from build123d import *

# Parameters (mm, degrees)
EXTRUDE_1_DEPTH     = 30
CUT_EXTRUDE_2_DEPTH = 60.044241887
EXTRUDE_2_DEPTH     = 30
FILLET_2_R          = 10
FILLET_3_R          = 10
SKETCH_6_R          = 1.65
CUT_EXTRUDE_3_DEPTH = 60.044242053
FILLET_4_R          = 2
FILLET_6_R          = 5


with BuildPart() as part:
    # 草图2 → 凸台-拉伸1 (new body)
    with BuildSketch(Plane.XY):
        with BuildLine():
            Line((-22, 40.85), (-22, -8.75))
            ThreePointArc((-22, -8.75), (-18.485281374, -17.235281374), (-10, -20.75))
            Line((-10, -20.75), (-10, -17.85))
            ThreePointArc((-10, -17.85), (-16.434671709, -15.184671709), (-19.1, -8.75))
            Line((-19.1, -8.75), (-19.1, 9.75))
            ThreePointArc((-19.1, 9.75), (-16.727564928, 15.477564928), (-11, 17.85))
            Line((-11, 17.85), (-5, 17.85))
            Line((-5, 17.85), (-5, 45.85))
            Line((-5, 45.85), (-17, 45.85))
            ThreePointArc((-17, 45.85), (-20.535533906, 44.385533906), (-22, 40.85))
        make_face()
    extrude(amount=EXTRUDE_1_DEPTH)

    # 草图4 → 切除-拉伸2 (cut, through all)
    with BuildSketch(Plane.XY.offset(30)):
        with BuildLine():
            Line((-10, -17.85), (-10, -20.75))
            ThreePointArc((-10, -20.75), (-14.258140623, -19.969101498), (-17.962085308, -17.728039739))
            ThreePointArc((-17.962085308, -17.728039739), (-15.915153532, -17.605278578), (-16.037914692, -15.558346802))
            ThreePointArc((-16.037914692, -15.558346802), (-13.229089973, -17.257818636), (-10, -17.85))
        make_face()
    extrude(amount=-CUT_EXTRUDE_2_DEPTH, mode=Mode.SUBTRACT)

    # 草图5 → 凸台-拉伸2 (add, through all)
    with BuildSketch(Plane.XY.offset(30)):
        with BuildLine():
            Line((-17.6, -8.75), (-19.1, -8.75))
            Line((-19.1, -8.75), (-19.1, -14.554532695))
            Line((-19.1, -14.554532695), (-15.915153532, -17.605278578))
            Line((-15.915153532, -17.605278578), (-14.952977082, -16.520329338))
            ThreePointArc((-14.952977082, -16.520329338), (-14.577681338, -15.439383984), (-15.073820173, -14.408299113))
            ThreePointArc((-15.073820173, -14.408299113), (-16.939777854, -11.848303301), (-17.6, -8.75))
        make_face()
    extrude(amount=-EXTRUDE_2_DEPTH)

    # 圆角2
    # the kernel refuses this fillet: 10 mm, written as the material it adds along each edge
    with BuildSketch(Plane(origin=(-19.1, -8.75, 0), x_dir=(0, 1, 0), z_dir=(0, 0, 1))) as fillet_2_piece_1:
        with BuildLine():
            CenterArc((5.267826876, -10), FILLET_2_R, 90, 31.788330617)
            Line((0, -1.5), (-0.105356538, -1.33))
            ThreePointArc((-0.105356538, -1.33), (-0.2, -0.75), (-0.2, 0))
            Line((-0.2, 0), (0, 0.2))
            Line((0, 0.2), (5.267826876, 0.2))
            Line((5.267826876, 0.2), (5.267826876, 0))
        make_face()
    extrude(amount=30)

    # 圆角3
    fillet_3_edges = [part.edges().sort_by_distance(p)[0] for p in [
        (-17.6, -8.75, 15),
    ]]
    fillet(fillet_3_edges, radius=FILLET_3_R)

    # 草图6 → 切除-拉伸3 (cut, through all)
    with BuildSketch(Plane.XY.offset(30)):
        with Locations((-8, 21.85)):
            Circle(SKETCH_6_R)
        with Locations((-18.301374289, 42.382296182)):
            Circle(SKETCH_6_R)
    extrude(amount=-CUT_EXTRUDE_3_DEPTH, mode=Mode.SUBTRACT)

    # 圆角4
    fillet_4_edges = [part.edges().sort_by_distance(p)[0] for p in [
        (-5, 17.85, 15),
    ]]
    fillet(fillet_4_edges, radius=FILLET_4_R)

    # 圆角6
    fillet_6_edges = [part.edges().sort_by_distance(p)[0] for p in [
        (-5, 45.85, 15),
    ]]
    fillet(fillet_6_edges, radius=FILLET_6_R)


solid = part.part
Geometry check sheet. Reference: the model listing, model coordinates, mm. A direction names the side the tool comes from. Give positions to 0.01 mm unless a question says otherwise; leave off trailing zeros. Write each loop counter-clockwise with the first axis right and the second up, starting at its lowest first coordinate (ties: lowest second). Pieces come first, ordered by that corner, then holes. Notation, with made-up numbers: M -35,58 L -21,58 A22 cw -21,86 Z; hole C 76.25,67 d8. An arc over 180 degrees is marked long. Answer as CSV lines item,"result". Start each with the question number.
Q1. Section check C-C, the plane z = 24.5. Give the number of separate pieces and of enclosed holes in the cut face, then the cut area to 3 significant figures.
Q2. Release check for a two-part mould opening along Y. For faces 4 (the face through (-18.516, 44.018, 15.21)), 5 (the face through (-18.886, -5.538, 14.79)), 6 (the face through (-5.6, 18.42, 15.21)), 7 (the face through (-6.43, 44.35, 15.21)) record: pulls with the +Y half, pulls with the -Y half, needs draft (parallel to the pull), parting line crosses it, or undercut.
Q3. Material ranges on L1, parallel to Y at x = -19.5, z = 12; L2, parallel to X at y = 9.5, z = 18.5; L3, parallel to Y at x = -8, z = 10, recorded low to high.
Q4. Section check B-B, the plane x = -8. Record the cut outline in (y, z), then the cut area to 3 significant figures.
Q5. Go/stop test with flat-tipped pins: pin 1 (5 mm diameter, centred on x = -7, z = 23.5, fed in from +Y); pin 2 (2 mm diameter, centred on x = -10, z = 12, fed in from -Y); pin 3 (10.5 mm diameter, centred on y = 4, z = 15.5, fed in from +X). Record where each tip stops, or that it passes through.
Q6. Section check A-A, the plane y = 21.85. Record the cut outline in (x, z), then the cut area to 3 significant figures.
Q7. Section check D-D, the plane x = -12. Record the cut outline in (y, z), then the cut area to 3 significant figures.
Q8. Tool access check on faces 1 (the face through (-16, 21, 30)), 2 (the face through (-16.644, -12.441, 15.21)), 3 (the face through (-9, 17.85, 15)). Record the directions out of +Z, -Z, +X, -X, +Y, -Y that give a thin tool (end or side, any length) a straight path to the whole face; none if there is none.
Geometry says:
1,separate pieces,"1"
1,enclosed holes,"2"
1,area,"583 mm^2"
2,face 4,"undercut"
2,face 5,"undercut"
2,face 6,"pulls with the -Y half"
2,face 7,"pulls with the +Y half"
3,L1,"-16.08 to 41.25, 43.52 to 45.18"
3,L2,"-22 to -19.1"
3,L3,"17.85 to 20.2, 23.5 to 45.43"
4,outline,"M 17.85,0 L 20.2,0 L 20.2,30 L 17.85,30 Z; M 23.5,0 L 45.43,0 L 45.43,30 L 23.5,30 Z"
4,area,"728 mm^2"
5,pin 1,"y = 45.82"
5,pin 2,"y = 17.85"
5,pin 3,"x = -19.1"
6,outline,"M -22,0 L -9.65,0 L -9.65,30 L -22,30 Z; M -6.35,0 L -5,0 L -5,30 L -6.35,30 Z"
6,area,"411 mm^2"
7,outline,"M 17.79,0 L 45.85,0 L 45.85,30 L 17.79,30 Z"
7,area,"842 mm^2"
8,face 1,"+Z, +X, -X, +Y, -Y"
8,face 2,"+Z, -Z, +X"
8,face 3,"+Z, -Z, +X, -Y"
